```python
from build123d import *

# Parameters (mm, degrees)
SKETCH1_R           = 19.812
SKETCH1_R_2         = 2.0828
BOSS_EXTRUDE1_DEPTH = 4.7625
BOSS_EXTRUDE2_DEPTH = 4.7625
FILLET1_R           = 2.54


with BuildPart() as part:
    # Sketch1 → Boss-Extrude1 (new body)
    with BuildSketch(Plane.XY):
        Polygon((-27.178, -30.226), (27.178, -30.226), (30.988, -26.416), (30.988, 39.878), (-30.988, 39.878), (-30.988, -26.416), align=None)
        with Locations(Location((0, 0, 0), (0, 0, 180))):
            Circle(SKETCH1_R, mode=Mode.SUBTRACT)
        with Locations(Location((-23.5712, 23.5712, 0), (0, 0, 180))):
            Circle(SKETCH1_R_2, mode=Mode.SUBTRACT)
        with Locations(Location((23.5712, 23.5712, 0), (0, 0, 180))):
            Circle(SKETCH1_R_2, mode=Mode.SUBTRACT)
        with Locations(Location((23.5712, -23.5712, 0), (0, 0, 180))):
            Circle(SKETCH1_R_2, mode=Mode.SUBTRACT)
        with Locations(Location((-23.5712, -23.5712, 0), (0, 0, 180))):
            Circle(SKETCH1_R_2, mode=Mode.SUBTRACT)
    extrude(amount=BOSS_EXTRUDE1_DEPTH)

    # Sketch4 → Boss-Extrude2 (add)
    with BuildSketch(Plane(origin=(0, 39.878, 0), x_dir=(-1, 0, 0), z_dir=(0, 1, 0))):
        with BuildLine():
            Line((12.7, 55.118), (41.656, 55.118))
            Line((41.656, 55.118), (41.656, 10.921672672))
            Line((41.656, 10.921672672), (30.988, 4.7625))
            Line((30.988, 4.7625), (30.988, 0))
            Line((30.988, 0), (-30.988, 0))
            Line((-30.988, 0), (-30.988, 4.7625))
            Line((-30.988, 4.7625), (-41.656, 10.921672672))
            Line((-41.656, 10.921672672), (-41.656, 55.118))
            Line((-41.656, 55.118), (-12.7, 55.118))
            Line((-12.7, 55.118), (-12.7, 42.418))
            ThreePointArc((-12.7, 42.418), (0, 29.718), (12.7, 42.418))
            Line((12.7, 42.418), (12.7, 55.118))
        make_face()
        with BuildLine():
            Line((-30.734, 47.117), (-37.338, 47.117))
            ThreePointArc((-37.338, 47.117), (-39.497, 44.958), (-37.338, 42.799))
            Line((-37.338, 42.799), (-30.734, 42.799))
            ThreePointArc((-30.734, 42.799), (-28.575, 44.958), (-30.734, 47.117))
        make_face(mode=Mode.SUBTRACT)
        with BuildLine():
            Line((-30.734, 21.717), (-37.338, 21.717))
            ThreePointArc((-37.338, 21.717), (-39.497, 19.558), (-37.338, 17.399))
            Line((-37.338, 17.399), (-30.734, 17.399))
            ThreePointArc((-30.734, 17.399), (-28.575, 19.558), (-30.734, 21.717))
        make_face(mode=Mode.SUBTRACT)
        with BuildLine():
            Line((37.338, 17.399), (30.734, 17.399))
            ThreePointArc((30.734, 17.399), (28.575, 19.558), (30.734, 21.717))
            Line((30.734, 21.717), (37.338, 21.717))
            ThreePointArc((37.338, 21.717), (39.497, 19.558), (37.338, 17.399))
        make_face(mode=Mode.SUBTRACT)
        with BuildLine():
            Line((37.338, 42.799), (30.734, 42.799))
            ThreePointArc((30.734, 42.799), (28.575, 44.958), (30.734, 47.117))
            Line((30.734, 47.117), (37.338, 47.117))
            ThreePointArc((37.338, 47.117), (39.497, 44.958), (37.338, 42.799))
        make_face(mode=Mode.SUBTRACT)
    extrude(amount=-BOSS_EXTRUDE2_DEPTH)

    # Fillet1
    fillet1_edges = [part.edges().sort_by_distance(p)[0] for p in [
        (0, 35.1155, 4.7625),
        (0, 39.878, 0),
    ]]
    fillet(fillet1_edges, radius=FILLET1_R)


solid = part.part
```
Input: part model. Units: mm. Frame: model coordinates. A direction names the side the tool comes from. Give positions to 0.01 mm unless a question says otherwise; leave off trailing zeros. Order: outer loops, then holes, each group sorted by start corner. A loop starts at its lowest first (then second) coordinate and runs counter-clockwise, first axis right, second up.
1. Mould query, pull axis Z, two halves, no side actions, for faces 1 (the flat face through (30.988, 6, 2)), 2 (the flat face through (-7, 19, 0)), 3 (the cylindrical face through (39.496, 37.53, 45.005)). Classes: released by +Z, released by -Z, zero draft, split by the parting line, or undercut.
Derived:
face 1: zero draft
face 2: released by -Z
face 3: undercut
2. Section D-D on y = 27. Return the cut outline in (x, z), and give its area (3 significant figures).
Derived:
outline: (-30.99, 0) - (30.99, 0) - (30.99, 4.76) - (-30.99, 4.76) - close
area: 295 mm2
3. Material intervals for L1, parallel to Y at x = 0, z = 2.7; L2, parallel to Z at x = 17, y = 15.5; L3, parallel to Y at x = 13.5, z = 42, sorted ascending.
Derived:
L1: y = -30.23 to -19.81, 19.81 to 39.88
L2: z = 0 to 4.76
L3: y = 35.12 to 39.88
4. Section C-C on y = -8. Return the cut outline in (x, z) (1 decimal).
Derived:
outline: (-31, 0) - (-18.1, 0) - (-18.1, 4.8) - (-31, 4.8) - close; (18.1, 0) - (31, 0) - (31, 4.8) - (18.1, 4.8) - close
5. Reachability of faces 4 (the flat face through (-14, 16, 4.762)), 5 (the flat face through (27, 38, 55.118)), 6 (the flat face through (34, 38, 21.717)) from +Z, -Z, +X, -X, +Y, -Y: full face, straight path, thin tool, end or side. Return the list, or none.
Derived:
face 4: +Z, +X, -X, -Y
face 5: +Z, +X, -X, +Y, -Y
face 6: +Y, -Y
6. Section A-A on x = 0. Return the cut outline in (y, z).
Derived:
outline: (-30.23, 0) - (-19.81, 0) - (-19.81, 4.76) - (-30.23, 4.76) - close; (19.81, 0) - (37.34, 0) arc R2.54 ccw to (39.88, 2.54) - (39.88, 29.72) - (35.12, 29.72) - (35.12, 7.3) arc R2.54 cw to (32.58, 4.76) - (19.81, 4.76) - close
7. Pin query (flat end, axial travel): pin 1 (2.5 mm diameter, centred on x = 35.5, y = 38.5, fed in from -Z); pin 2 (5 mm diameter, centred on x = 34, y = 36.5, fed in from -Z); pin 3 (6 mm diameter, centred on x = 8, z = 20.5, fed in from -Y). Return the tip coordinate at first contact, or that it passes through.
Derived:
pin 1: stops at z = 6.65
pin 2: stops at z = 5.06
pin 3: stops at y = 35.12
8. Section B-B on y = 0. Return the cut outline in (x, z), and give its area (3 significant figures).
Derived:
outline: (-30.99, 0) - (-19.81, 0) - (-19.81, 4.76) - (-30.99, 4.76) - close; (19.81, 0) - (30.99, 0) - (30.99, 4.76) - (19.81, 4.76) - close
area: 106 mm2
